Work out the finished part from the listing and answer in its coordinate system (mm). A direction names the side the tool comes from. Round coordinates to 2 decimals unless told otherwise and drop trailing zeros. Order: outer loops, then holes, each group sorted by start corner. A loop starts at its lowest first (then second) coordinate and runs counter-clockwise, first axis right, second up. Notation, with made-up numbers: M 11,41 L 63,41 A21 cw 63,46 Z; hole C -7.5,15 d11. An arc over 180 degrees is marked long. Answer as a JSON object with one key per item and string values. Group by question number.
Autodesk Inventor part; units mm, degrees
ref_plane "YZ Plane" through (0, 0, 0) normal (1, 0, 0) x (0, 1, 0)
ref_plane "XZ Plane" through (0, 0, 0) normal (0, 1, 0) x (-1, 0, 0)
ref_plane "XY Plane" through (0, 0, 0) normal (0, 0, 1) x (1, 0, 0)
sketch "Sketch1" plane through (0, 0, 0) normal (0, 0, 1) x (1, 0, 0)
  line L0 (86, 6) -> (86, 106)
  line L1 (2021.3603, 237.2065) -> (2021.3603, 237.2065) construction
  arc A0 (80, 0) -> (86, 6) centre (80, 6) ccw
  line L2 (0, 0) -> (80, 0)
  dimension "d25" = 6
  dimension "d46" = 90
  dimension "d47" = 80
  dimension "d48" = 100
contour flange "Contour Flange1" sketch "Sketch1" thickness 3 bend radius 3 width 2700 along (0, 0, 1) mid plane no both sides no wall seen from (40, 0, 0) lies toward (0, 1, 0) curves L2 A0 L0
bend "Bend1"
corner "Corner1"
mirror "Mirror1" about plane through (0, 0, 0) normal (1, 0, 0)
equation "\"d25\" = Thickness + BendRadius"
equation "\"d7\" = Thickness"
equation "\"d8\" = BendReliefWidth"
equation "\"d9\" = BendReliefDepth"
equation "\"d10\" = MinimumRemnant"
equation "\"d11\" = TransitionRadius"
equation "\"d13\" = BendRadius"
equation "\"d15\" = CornerReliefSize"
equation "\"d16\" = GapSize"
equation "\"d17\" = JacobiRadiusSize"
equation "\"BendRadius\" = Thickness"
equation "\"BendReliefWidth\" = Thickness"
equation "\"BendReliefDepth\" = 0.5 * Thickness"
equation "\"CornerReliefSize\" = 4 * Thickness"
equation "\"MinimumRemnant\" = 2 * Thickness"
equation "\"TransitionRadius\" = BendRadius"
equation "\"JacobiRadiusSize\" = BendRadius"
equation "\"GapSize\" = Thickness"
equation "\"d38\" = d40 + d44"
equation "\"d39\" = d40"
equation "\"d44\" = d40"
properties part number "MSC 077 screen pillar" material "Stainless Steel"
Item 1: This flat-tipped pin is pushed along its axis until it touches: pin 1 (1.5 mm diameter, centred on x = -63, z = 573.5, fed in from +Y). Where does it stop, or does it pass through?
Item 2: Find section C-C (x = -0.5). Give the vertices of the cut face in (y, z).
Item 3: A tool of negligible diameter and unlimited length cuts with its end or side. For faces 1 (the flat face through (86, 55, 1331)), 2 (the flat face through (-83, 57, 1331)), from which of +Z, -Z, +X, -X, +Y, -Y can it reach the whole face along a straight path? Write none if from no direction.
Item 4: The mould has two halves that part along X. Classify faces 3 (the flat face through (-86, 57, 1331)), 4 (the flat face through (-1, 3, 1331)), 5 (the flat face through (83, 55, 1331)), 6 (the flat face through (-39, 2, 2700)): +X half, -X half, draft (parallel to the pull), parting line (faces both ways), or undercut.
Item 5: Find section B-B (z = 1711.5). Give the vertices of the cut face in (x, y).
Item 6: Find section A-A (y = 81.5). Give the vertices of the cut face in (x, z).
Item 7: Consider L1, parallel to X at y = 38, z = 418; L2, parallel to Y at x = 22.5, z = 189. Determine where each line is inside the solid, lowest interval first.
Responses:
{
 "1": {"pin 1": "stops at y = 3"},
 "2": {"outline": "M 0,0 L 3,0 L 3,2700 L 0,2700 Z"},
 "3": {"face 1": "+Z, -Z, +X, +Y, -Y", "face 2": "+Z, -Z, +Y"},
 "4": {"face 3": "-X half", "face 4": "undercut", "face 5": "undercut", "face 6": "draft"},
 "5": {"outline": "M -86,6 A6 ccw -80,0 L 80,0 A6 ccw 86,6 L 86,106 L 83,106 L 83,6 A3 cw 80,3 L -80,3 A3 cw -83,6 L -83,106 L -86,106 Z"},
 "6": {"outline": "M -86,0 L -83,0 L -83,2700 L -86,2700 Z; M 83,0 L 86,0 L 86,2700 L 83,2700 Z"},
 "7": {"L1": "x = -86 to -83, 83 to 86", "L2": "y = 0 to 3"}
}
